```python
from build123d import *

# Parameters (mm, degrees)
F0_R     = 45
F1_DEPTH = 15
F2_W     = 47.7026963846
F2_H     = 45
F5_F1_R  = 5
F5_F2_R  = 5


with BuildPart() as f1:
    # F0 (on Right) → F1 (new body)
    with BuildSketch(Plane.YZ):
        Circle(F0_R)
    extrude(amount=F1_DEPTH)

    # F4: sweep along a path in F3
    with BuildLine(Plane.XZ) as f4_path:
        Line((15, 0), (80, 0))
        ThreePointArc((80, 0), (122.4264068712, -17.5735931288), (140, -60))
        Line((140, -60), (140, -220))
        ThreePointArc((140, -220), (131.2132034356, -241.2132034356), (110, -250))
        Line((110, -250), (85, -250))
        ThreePointArc((85, -250), (63.7867965644, -258.7867965644), (55, -280))
        Line((55, -280), (55, -550))
    # F2 (on face) → F4 (sweep)
    with BuildSketch(Plane.YZ.offset(15)):
        Rectangle(F2_W, F2_H)
    sweep(path=f4_path.line)

    # F5: fillet of radius 5 on 34 edges, made by hand

    # F5_f1
    f5_f1_edges = [f1.edges().sort_by_distance(p)[0] for p in [
        (47.5, -23.8513481923, 22.5),
        (47.5, -23.8513481923, -22.5),
        (106.5165042945, -23.8513481923, -33.4834957055),
        (117.5, -23.8513481923, -140),
        (115.3033008589, -23.8513481923, -225.3033008589),
        (97.5, -23.8513481923, -227.5),
        (47.8768939877, -23.8513481923, -242.8768939877),
        (32.5, -23.8513481923, -415),
        (55, -23.8513481923, -550),
        (77.5, -23.8513481923, -415),
        (79.6966991411, -23.8513481923, -274.6966991411),
        (97.5, -23.8513481923, -272.5),
        (147.1231060123, -23.8513481923, -257.1231060123),
        (162.5, -23.8513481923, -140),
        (138.3363094479, -23.8513481923, -1.6636905521),
        (47.5, 23.8513481923, -22.5),
        (47.5, 23.8513481923, 22.5),
        (138.3363094479, 23.8513481923, -1.6636905521),
        (162.5, 23.8513481923, -140),
        (147.1231060123, 23.8513481923, -257.1231060123),
        (97.5, 23.8513481923, -272.5),
        (79.6966991411, 23.8513481923, -274.6966991411),
        (77.5, 23.8513481923, -415),
        (55, 23.8513481923, -550),
        (32.5, 23.8513481923, -415),
        (47.8768939877, 23.8513481923, -242.8768939877),
        (97.5, 23.8513481923, -227.5),
        (115.3033008589, 23.8513481923, -225.3033008589),
        (117.5, 23.8513481923, -140),
        (106.5165042945, 23.8513481923, -33.4834957055),
        (32.5, 0, -550),
        (77.5, 0, -550),
    ]]
    fillet(f5_f1_edges, radius=F5_F1_R)

    # F5_f2
    f5_f2_edges = [f1.edges().sort_by_distance(p)[0] for p in [
        (15, -23.8513481923, 0),
        (15, 23.8513481923, 0),
        (15, 22.3868820983, -21.0355339059),
        (15, 22.3868820983, 21.0355339059),
        (15, -22.3868820983, 21.0355339059),
        (15, -22.3868820983, -21.0355339059),
    ]]
    fillet(f5_f2_edges, radius=F5_F2_R)


solid = f1.part
```
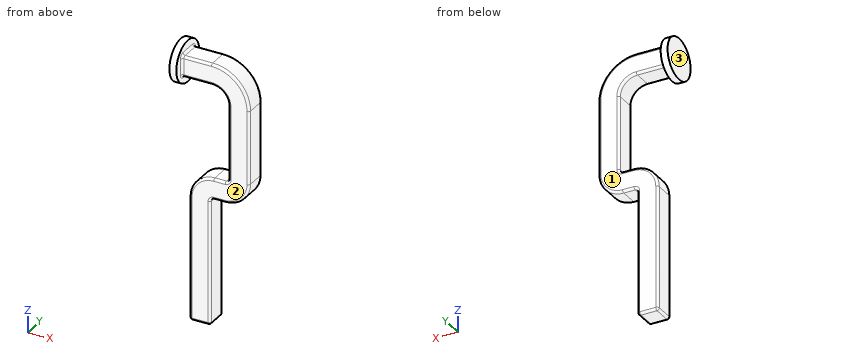
Design review of the part built by this model. Coordinates are the model's own, in mm. Face numbers are marked on the shaded views. A direction names the side the tool comes from. Round coordinates to 2 decimals unless told otherwise and drop trailing zeros. Write each loop counter-clockwise with the first axis right and the second up, starting at its lowest first coordinate (ties: lowest second). Pieces come first, ordered by that corner, then holes. Notation, with made-up numbers: (84, 85.5) -> (135, 85.5) arc R19 ccw to (135, 92.5) -> close; hole circle Ø2 at (89.25, 3.25). An arc over 180 degrees is marked (long way). Write item = value, one per line. Start each with the question number.
1) Take a section at A-A, the plane z = -380. State the section outline as (x, y) points, plus the area to 3 significant figures.
2) Tool access review of the marked faces 1, 2 and 3: name each direction out of +Z, -Z, +X, -X, +Y, -Y from which nothing blocks a thin tool from reaching the whole face with its end or side.
3) Take a section at B-B, the plane y = 0. State the section outline as (x, z) points, plus the area to 3 significant figures.
4) Wall thickness on probe 1 along Z at (x, y) = (69, -20); probe 2 along Z at (x, y) = (41, -13); probe 3 along Y at (x, z) = (41, -441.5): over which ranges is each line inside the solid? List them lowest first. Write a range as from..to.
5) Clearance check with flat-ended pins moving along their axes: pin 1 (8 mm diameter, centred on x = 133.5, z = -95.5, fed in from +Y); pin 2 (1 mm diameter, centred on x = 57.5, z = -439.5, fed in from -Y); pin 3 (11.5 mm diameter, centred on x = 37, y = 7.5, fed in from +Z). State where each tip first meets the part, or that it passes through.
Results list:
q1.outline = (32.5, -18.85) arc R5 ccw to (37.5, -23.85) -> (72.5, -23.85) arc R5 ccw to (77.5, -18.85) -> (77.5, 18.85) arc R5 ccw to (72.5, 23.85) -> (37.5, 23.85) arc R5 ccw to (32.5, 18.85) -> close
q1.area = 2,130 mm²
q2.face_1 = +Z, -Z, +X, +Y
q2.face_2 = +Z, -Z, +X, -Y
q2.face_3 = +Z, -Z, -X, +Y, -Y
q3.outline = (0, -45) -> (15, -45) -> (15, -27.5) arc R5 cw to (20, -22.5) -> (80, -22.5) arc R37.5 cw to (117.5, -60) -> (117.5, -220) arc R7.5 cw to (110, -227.5) -> (85, -227.5) arc R52.5 ccw to (32.5, -280) -> (32.5, -545) arc R5 ccw to (37.5, -550) -> (72.5, -550) arc R5 ccw to (77.5, -545) -> (77.5, -280) arc R7.5 cw to (85, -272.5) -> (110, -272.5) arc R52.5 ccw to (162.5, -220) -> (162.5, -60) arc R82.5 ccw to (80, 22.5) -> (20, 22.5) arc R5 cw to (15, 27.5) -> (15, 45) -> (0, 45) -> close
q3.area = 33,200 mm²
q4.probe_1 = -549.87..-230.14, -22.37..22.37
q4.probe_2 = -550..-251.36, -22.5..22.5
q4.probe_3 = -23.85..23.85
q5.pin_1 = 23.85
q5.pin_2 = -23.85
q5.pin_3 = 22.5
